Could you check a few things on this model? Use its own coordinates, in mm. Face numbers are marked on the shaded views. A direction names the side the tool comes from. Coordinates: 2 decimals unless noted, no trailing zeros. Loops run counter-clockwise (first coordinate to the right, second up) from the corner with the lowest first, then second, coordinate; pieces in that order, holes last.
1) Imagine slicing it at B-B on x = 7. Please give me the cut outline in (y, z).
2) Imagine slicing it at C-C on z = 6. Give the number of separate pieces and of enclosed holes in the cut face, plus the area to 3 significant figures.
3) For the marked faces 1 and 2, which set-ups out of +Z, -Z, +X, -X, +Y, -Y let a thin tool reach every point of the face, with its end or its side?
4) If I drill on line 1 along X through (y, z) = (34.5, 16.5); line 2 along X through (y, z) = (68.5, 24); line 3 along Y through (x, z) = (14.5, 14.75), over which ranges is the centre line in solid material (lowest first)?
5) Thinking about a two-plate mould opening in Y: for the marked faces 3, 4 and 5, which applies, released by +Y, released by -Y, zero draft, split by the parting line, or undercut?
6) Imagine slicing it at D-D on y = -92. Please give me the cut outline in (x, z).
7) Imagine slicing it at A-A on y = 41.5. Please give me the cut outline in (x, z), plus the area to 3 significant figures.
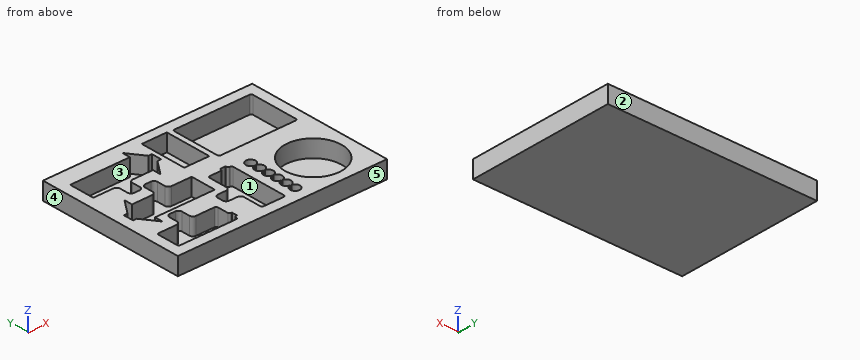
```python
from build123d import *

# Parameters (mm, degrees)
F0_W      = 304.8
F0_H      = 215.9
F1_DEPTH  = 25.4
F5_R      = 41.275
F8_W      = 36.5
F8_H      = 68
F10_DEPTH = 25


with BuildPart() as f1:
    # F0 (on Top) → F1 (new body)
    with BuildSketch(Plane.XY):
        with Locations((17.103421, -21.658359)):
            Rectangle(F0_W, F0_H)
    extrude(amount=F1_DEPTH)

    # F0 (on Top) + F2 (on face) + F3 (on face) + F4 (on face) + F5 (on face) + F6 (on face) + F7 (on face) + F8 (on face) + F9 (on face) → F10 (cut)
    with BuildSketch(Plane.XY):
        with Locations((17.103421, -21.658359)):
            Rectangle(F0_W, F0_H)
    with BuildSketch(Plane.XY.offset(25.4)):
        with BuildLine():
            Line((1.455991, -85.278079), (1.455991, -111.389279))
            ThreePointArc((1.455991, -111.389279), (2.19994, -113.18533), (3.995991, -113.929279))
            Line((3.995991, -113.929279), (33.459991, -113.929279))
            ThreePointArc((33.459991, -113.929279), (35.256042, -113.18533), (35.999991, -111.389279))
            Line((35.999991, -111.389279), (35.999991, -30.109279))
            ThreePointArc((35.999991, -30.109279), (35.256042, -28.313228), (33.459991, -27.569279))
            Line((33.459991, -27.569279), (33.129791, -27.569279))
            ThreePointArc((33.129791, -27.569279), (31.297819, -26.810451), (30.538991, -24.978479))
            Line((30.538991, -24.978479), (30.538991, -23.759279))
            Line((30.538991, -23.759279), (22.410991, -23.759279))
            Line((22.410991, -23.759279), (22.410991, -24.978479))
            ThreePointArc((22.410991, -24.978479), (21.652163, -26.810451), (19.820191, -27.569279))
            Line((19.820191, -27.569279), (3.995991, -27.569279))
            ThreePointArc((3.995991, -27.569279), (2.19994, -28.313228), (1.455991, -30.109279))
            Line((1.455991, -30.109279), (1.455991, -57.236479))
            ThreePointArc((1.455991, -57.236479), (-0.009588, -60.7747), (-3.547809, -62.240279))
            Line((-3.547809, -62.240279), (-15.536609, -62.240279))
            ThreePointArc((-15.536609, -62.240279), (-19.07483, -63.705858), (-20.540409, -67.244079))
            Line((-20.540409, -67.244079), (-20.540409, -75.270479))
            ThreePointArc((-20.540409, -75.270479), (-19.07483, -78.8087), (-15.536609, -80.274279))
            Line((-15.536609, -80.274279), (-3.547809, -80.274279))
            ThreePointArc((-3.547809, -80.274279), (-0.009588, -81.739858), (1.455991, -85.278079))
        make_face()
    with BuildSketch(Plane.XY.offset(25.4)):
        with BuildLine():
            Line((-98.282373, -52.532049), (-11.282373, -52.532049))
            Line((-11.282373, -52.532049), (-11.282373, -15.532049))
            Line((-11.282373, -15.532049), (-40.782373, -15.532049))
            ThreePointArc((-40.782373, -15.532049), (-44.317906, -14.067583), (-45.782373, -10.532049))
            Line((-45.782373, -10.532049), (-45.782373, 1.467951))
            ThreePointArc((-45.782373, 1.467951), (-47.246839, 5.003485), (-50.782373, 6.467951))
            Line((-50.782373, 6.467951), (-58.782373, 6.467951))
            ThreePointArc((-58.782373, 6.467951), (-62.317906, 5.003485), (-63.782373, 1.467951))
            Line((-63.782373, 1.467951), (-63.782373, -10.532049))
            ThreePointArc((-63.782373, -10.532049), (-65.246839, -14.067583), (-68.782373, -15.532049))
            Line((-68.782373, -15.532049), (-98.282373, -15.532049))
            Line((-98.282373, -15.532049), (-98.282373, -3.532049))
            Line((-98.282373, -3.532049), (-114.939746, -26.682049))
            Line((-114.939746, -26.682049), (-120.228373, -26.682049))
            Line((-120.228373, -26.682049), (-120.228373, -34.032049))
            Line((-120.228373, -34.032049), (-120.228373, -41.382049))
            Line((-120.228373, -41.382049), (-114.939746, -41.382049))
            Line((-114.939746, -41.382049), (-98.282373, -64.532049))
            Line((-98.282373, -64.532049), (-98.282373, -52.532049))
        make_face()
    with BuildSketch(Plane.XY.offset(25.4)):
        with BuildLine():
            Line((151.751869, 70.914), (42.277869, 70.914))
            ThreePointArc((42.277869, 70.914), (40.481818, 70.170051), (39.737869, 68.374))
            Line((39.737869, 68.374), (39.737869, -0.46))
            ThreePointArc((39.737869, -0.46), (40.481818, -2.256051), (42.277869, -3))
            Line((42.277869, -3), (151.751869, -3))
            ThreePointArc((151.751869, -3), (153.54792, -2.256051), (154.291869, -0.46))
            Line((154.291869, -0.46), (154.291869, 68.374))
            ThreePointArc((154.291869, 68.374), (153.54792, 70.170051), (151.751869, 70.914))
        make_face()
    with BuildSketch(Plane.XY.offset(25.4)):
        with Locations((112.600401, -74.001856)):
            Circle(F5_R)
    with BuildSketch(Plane.XY.offset(25.4)):
        with BuildLine():
            Line((-91.696568, -79.872966), (-117.807768, -79.872966))
            ThreePointArc((-117.807768, -79.872966), (-119.603819, -80.616915), (-120.347768, -82.412966))
            Line((-120.347768, -82.412966), (-120.347768, -111.876966))
            ThreePointArc((-120.347768, -111.876966), (-119.603819, -113.673017), (-117.807768, -114.416966))
            Line((-117.807768, -114.416966), (-36.527768, -114.416966))
            ThreePointArc((-36.527768, -114.416966), (-34.731717, -113.673017), (-33.987768, -111.876966))
            Line((-33.987768, -111.876966), (-33.987768, -111.546766))
            ThreePointArc((-33.987768, -111.546766), (-33.22894, -109.714794), (-31.396968, -108.955966))
            Line((-31.396968, -108.955966), (-30.177768, -108.955966))
            Line((-30.177768, -108.955966), (-30.177768, -100.827966))
            Line((-30.177768, -100.827966), (-31.396968, -100.827966))
            ThreePointArc((-31.396968, -100.827966), (-33.22894, -100.069138), (-33.987768, -98.237166))
            Line((-33.987768, -98.237166), (-33.987768, -82.412966))
            ThreePointArc((-33.987768, -82.412966), (-34.731717, -80.616915), (-36.527768, -79.872966))
            Line((-36.527768, -79.872966), (-63.654968, -79.872966))
            ThreePointArc((-63.654968, -79.872966), (-67.193189, -78.407387), (-68.658768, -74.869166))
            Line((-68.658768, -74.869166), (-68.658768, -62.880366))
            ThreePointArc((-68.658768, -62.880366), (-70.124347, -59.342145), (-73.662568, -57.876566))
            Line((-73.662568, -57.876566), (-81.688968, -57.876566))
            ThreePointArc((-81.688968, -57.876566), (-85.227189, -59.342145), (-86.692768, -62.880366))
            Line((-86.692768, -62.880366), (-86.692768, -74.869166))
            ThreePointArc((-86.692768, -74.869166), (-88.158347, -78.407387), (-91.696568, -79.872966))
        make_face()
    with BuildSketch(Plane.XY.offset(25.4)):
        with BuildLine():
            Line((56.581123, -43.780106), (56.581123, -43.537542))
            ThreePointArc((56.581123, -43.537542), (55.581123, -29.508824), (54.581123, -43.537542))
            Line((54.581123, -43.537542), (54.581123, -43.780106))
            ThreePointArc((54.581123, -43.780106), (48.531123, -50.758824), (54.581123, -57.737542))
            Line((54.581123, -57.737542), (54.581123, -57.980106))
            ThreePointArc((54.581123, -57.980106), (48.531123, -64.958824), (54.581123, -71.937542))
            Line((54.581123, -71.937542), (54.581123, -72.180106))
            ThreePointArc((54.581123, -72.180106), (48.531123, -79.158824), (54.581123, -86.137542))
            Line((54.581123, -86.137542), (54.581123, -86.380106))
            ThreePointArc((54.581123, -86.380106), (48.531123, -93.358824), (54.581123, -100.337542))
            Line((54.581123, -100.337542), (54.581123, -100.580106))
            ThreePointArc((54.581123, -100.580106), (55.581123, -114.608824), (56.581123, -100.580106))
            Line((56.581123, -100.580106), (56.581123, -100.337542))
            ThreePointArc((56.581123, -100.337542), (62.631123, -93.358824), (56.581123, -86.380106))
            Line((56.581123, -86.380106), (56.581123, -86.137542))
            ThreePointArc((56.581123, -86.137542), (62.631123, -79.158824), (56.581123, -72.180106))
            Line((56.581123, -72.180106), (56.581123, -71.937542))
            ThreePointArc((56.581123, -71.937542), (62.631123, -64.958824), (56.581123, -57.980106))
            Line((56.581123, -57.980106), (56.581123, -57.737542))
            ThreePointArc((56.581123, -57.737542), (62.631123, -50.758824), (56.581123, -43.780106))
        make_face()
    with BuildSketch(Plane.XY.offset(25.4)):
        with Locations((13.897042, 38)):
            Rectangle(F8_W, F8_H)
    with BuildSketch(Plane.XY.offset(25.4)):
        with BuildLine():
            Line((-32.676903, 59.959536), (-119.676903, 59.959536))
            Line((-119.676903, 59.959536), (-119.676903, 22.959536))
            Line((-119.676903, 22.959536), (-90.176903, 22.959536))
            ThreePointArc((-90.176903, 22.959536), (-86.641369, 21.49507), (-85.176903, 17.959536))
            Line((-85.176903, 17.959536), (-85.176903, 5.959536))
            ThreePointArc((-85.176903, 5.959536), (-83.712437, 2.424002), (-80.176903, 0.959536))
            Line((-80.176903, 0.959536), (-72.176903, 0.959536))
            ThreePointArc((-72.176903, 0.959536), (-68.641369, 2.424002), (-67.176903, 5.959536))
            Line((-67.176903, 5.959536), (-67.176903, 17.959536))
            ThreePointArc((-67.176903, 17.959536), (-65.712437, 21.49507), (-62.176903, 22.959536))
            Line((-62.176903, 22.959536), (-32.676903, 22.959536))
            Line((-32.676903, 22.959536), (-32.676903, 10.959536))
            Line((-32.676903, 10.959536), (-16.019529, 34.109536))
            Line((-16.019529, 34.109536), (-10.730903, 34.109536))
            Line((-10.730903, 34.109536), (-10.730903, 41.459536))
            Line((-10.730903, 41.459536), (-10.730903, 48.809536))
            Line((-10.730903, 48.809536), (-16.019529, 48.809536))
            Line((-16.019529, 48.809536), (-32.676903, 71.959536))
            Line((-32.676903, 71.959536), (-32.676903, 59.959536))
        make_face()
    extrude(amount=-F10_DEPTH, mode=Mode.SUBTRACT)


solid = f1.part
```
Filled in:
1. outline: (-129.61, 0) - (86.29, 0) - (86.29, 25.4) - (72, 25.4) - (72, 0.4) - (4, 0.4) - (4, 25.4) - (-27.57, 25.4) - (-27.57, 0.4) - (-113.93, 0.4) - (-113.93, 25.4) - (-129.61, 25.4) - close
2. separate pieces: 1
2. enclosed holes: 8
2. area: 33,100 mm2
3. face 1: +Z
3. face 2: +Z, -Z, +X, -X, +Y
4. line 1: x = -135.3 to -119.68, -10.73 to -4.35, 32.15 to 39.74, 154.29 to 169.5
4. line 2: x = -135.3 to -32.68, -30.19 to -4.35, 32.15 to 39.74, 154.29 to 169.5
4. line 3: y = -129.61 to -113.93, -27.57 to 4, 72 to 86.29
5. face 3: undercut
5. face 4: zero draft
5. face 5: released by -Y
6. outline: (-135.3, 0) - (169.5, 0) - (169.5, 25.4) - (149.74, 25.4) - (149.74, 0.4) - (75.46, 0.4) - (75.46, 25.4) - (62.5, 25.4) - (62.5, 0.4) - (48.66, 0.4) - (48.66, 25.4) - (36, 25.4) - (36, 0.4) - (1.46, 0.4) - (1.46, 25.4) - (-33.99, 25.4) - (-33.99, 0.4) - (-120.35, 0.4) - (-120.35, 25.4) - (-135.3, 25.4) - close
7. outline: (-135.3, 0) - (169.5, 0) - (169.5, 25.4) - (154.29, 25.4) - (154.29, 0.4) - (39.74, 0.4) - (39.74, 25.4) - (32.15, 25.4) - (32.15, 0.4) - (-4.35, 0.4) - (-4.35, 25.4) - (-10.73, 25.4) - (-10.73, 0.4) - (-119.68, 0.4) - (-119.68, 25.4) - (-135.3, 25.4) - close
7. area: 1,240 mm2
